Work out the finished part from the listing and answer in its coordinate system (mm). Face numbers are marked on the shaded views. A direction names the side the tool comes from. Give positions to 0.01 mm unless a question says otherwise; leave off trailing zeros. Loops run counter-clockwise (first coordinate to the right, second up) from the corner with the lowest first, then second, coordinate; pieces in that order, holes last. Notation, with made-up numbers: (16.5, 0.25) - (43.5, 0.25) arc R18 ccw to (43.5, 17.25) - close; hole circle Ø5 at (4.5, 47.25). An arc over 180 degrees is marked (long way). One line per question, with ' | ' between items.
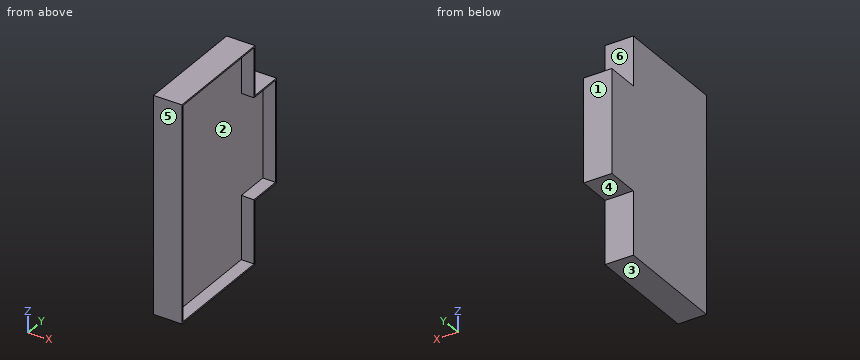
from build123d import *

# Parameters (mm, degrees)
F0_W     = 111.8879971261
F0_H     = 182.8464864036
F0_W_2   = 58.7416736197
F1_DEPTH = 50
F2_T     = -2.54
F3_DEPTH = 25
F4_R     = 48.7363148041
F5_DEPTH = 25
F6_DEPTH = 25


with BuildPart() as f1:
    # F0 (on Right) → F1 (new body)
    with BuildSketch(Plane.YZ):
        Polygon((0, -93.3897359272), (0, 89.4567504763), (111.8879971261, 89.4567504763), (111.8879971261, 176.4833948933), (-88.1120028739, 176.4833948933), (-88.1120028739, -205.3286014106), (111.8879971261, -205.3286014106), (111.8879971261, -93.3897359272), align=None)
        with Locations((55.9439985631, -1.9664927255)):
            Rectangle(F0_W, F0_H)
        with Locations((141.258833936, -1.9664927255)):
            Rectangle(F0_W_2, F0_H)
    extrude(amount=F1_DEPTH)

    # F2
    f2_openings = [f1.faces().sort_by_distance(p)[0] for p in [
        (50, 27.840751, -12.886637),
    ]]
    offset(amount=F2_T, openings=f2_openings, kind=Kind.INTERSECTION)

    # F3 (add): a face of the model
    f3_faces = [f1.faces().sort_by_distance(p)[0] for p in [
        (2.54, 27.6782483044, -12.8718359613),
    ]]
    extrude(f3_faces, amount=F3_DEPTH)

    # F4 (on face) → F5 (join)
    with BuildSketch(Plane.YZ.offset(27.54)):
        Circle(F4_R)
    extrude(amount=F5_DEPTH)

    # F6 (cut): a face of the model
    f6_faces = [f1.faces().sort_by_distance(p)[0] for p in [
        (52.54, 0, 0),
    ]]
    extrude(f6_faces, amount=-F6_DEPTH, mode=Mode.SUBTRACT)


solid = f1.part
1. Which of the six approach directions +Z, -Z, +X, -X, +Y, -Y give full straight-line access (tool end or side, diameter ignored) to the marked faces 4, 5 and 6?
Evaluation:
face 4: -Z, +X, -X, +Y | face 5: +Z, -Z, +X, -X, -Y | face 6: +Z, +X, -X, +Y
2. Find section C-C on x = 42. Write down the section's boundary in (y, z), then the cut area to 3 significant figures.
Evaluation:
outline: (-88.11, -205.33) - (111.89, -205.33) - (111.89, -93.39) - (170.63, -93.39) - (170.63, 89.46) - (111.89, 89.46) - (111.89, 176.48) - (-88.11, 176.48) - close; hole (-85.57, -202.79) - (109.35, -202.79) - (109.35, -90.85) - (168.09, -90.85) - (168.09, 86.92) - (109.35, 86.92) - (109.35, 173.94) - (-85.57, 173.94) - close | area: 3,230 mm2
3. Find section A-A on z = 64.5. Write down the section's boundary in (x, y).
Evaluation:
outline: (0, -88.11) - (50, -88.11) - (50, -85.57) - (27.54, -85.57) - (27.54, 168.09) - (50, 168.09) - (50, 170.63) - (0, 170.63) - close
4. Consider L1, parallel to Z at x = 42.5, y = 23; L2, parallel to Y at x = 36, z = -66.5; L3, parallel to Y at x = 39.5, z = -160. Determine where each line is inside the solid, lowest interval first.
Evaluation:
L1: -205.33 to -202.79, 173.94 to 176.48 | L2: -88.11 to -85.57, 168.09 to 170.63 | L3: -88.11 to -85.57, 109.35 to 111.89
5. Find section B-B on y = 143.5. Write down the section's boundary in (x, z), then the cut area to 3 significant figures.
Evaluation:
outline: (0, -93.39) - (50, -93.39) - (50, -90.85) - (27.54, -90.85) - (27.54, 86.92) - (50, 86.92) - (50, 89.46) - (0, 89.46) - close | area: 5,150 mm2
6. Flat-ended cylindrical pins translate along their axes: pin 1 (15 mm diameter, centred on x = 14, z = 117, fed in from +Y); pin 2 (4 mm diameter, centred on y = 67.5, z = 83.5, fed in from +X); pin 3 (25 mm diameter, centred on x = 33, y = 130.5, fed in from -Z). Find the tip coordinate at first contact, or state that the pin passes through.
Evaluation:
pin 1: y = 111.89 | pin 2: x = 27.54 | pin 3: z = -93.39
7. Determine the mould class of the marked faces 1, 2 and 3 for opening direction Z: +Z half, -Z half, draft (parallel to the pull), parting line (faces both ways), or undercut.
Evaluation:
face 1: draft | face 2: undercut | face 3: -Z half
